The model under review builds one solid part; all positions refer to its coordinate system, in mm. A direction names the side the tool comes from. Round coordinates to 2 decimals unless told otherwise and drop trailing zeros. Order: outer loops, then holes, each group sorted by start corner. A loop starts at its lowest first (then second) coordinate and runs counter-clockwise, first axis right, second up. Notation, with made-up numbers: (-27, 75) - (3, 75) arc R16 cw to (3, 88) - close; hole circle Ø7 at (56.5, -3.75). An arc over 180 degrees is marked (long way). One line per question, with ' | ' between items. Start each with the question number.
Item 1: Add section C-C on z = -13. State the section outline as (x, y) points, and give its area (3 significant figures).
Item 2: Add section B-B on x = 36. State the section outline as (y, z) points.
Item 3: Add section D-D on y = 40. State the section outline as (x, z) points.
Item 4: Draft analysis for pull direction Y (two halves, no side actions). For faces 3 (the face through (6.47, 27.98, -6.56)), 4 (the face through (1.43, 94.08, -51.93)), 5 (the face through (101, 52, -19)), 6 (the face through (51.2, 12.6, 4.4)), state which applies: +Y half, -Y half, draft (parallel to the pull), parting line (faces both ways), or undercut.
Item 5: Insertion check: pin 1 Ø7.5 at (x, y) = (31, 5) entering from -Z; pin 2 Ø3 at (x, y) = (6, 5) entering from +Z; pin 3 Ø1.5 at (x, y) = (23, 18.5) entering from -Z; pin 4 Ø10 at (x, z) = (82.5, -0.5) entering from -Y. Each pin has a flat end and moves straight along its axis. Give the tip position at first contact, or say it passes through.
Item 6: For L1, parallel to Y at x = 60.5, z = -32; L2, parallel to Y at x = 6, z = 1.35; L3, parallel to Z at x = 25, y = 17.5, list the stretches that pass through material, from the lowest coordinate up. Write a range as [from, to].
Item 7: Tool access review of faces 1 (the face through (10.07, 23.49, 17.67)), 2 (the face through (49.793, 94.212, -49.2)): name each direction out of +Z, -Z, +X, -X, +Y, -Y from which nothing blocks a thin tool from reaching the whole face with its end or side.
Item 8: Add section A-A on y = 19. State the section outline as (x, z) points, and give its area (3 significant figures).
from build123d import *

# Parameters (mm, degrees)
SKETCH_1_W               = 101
SKETCH_1_H               = 15
SKETCH_1_R               = 1.55
EXTRUDE_1_DEPTH          = 3
EXTRUDE_2_DEPTH          = 101
FILLET_1_R               = 10
FILLET_2_R               = 5
SKETCH_3_W               = 101
SKETCH_3_H               = 3
EXTRUDE_3_DEPTH          = 41
SKETCH_4_R               = 1.55
CUT_EXTRUDE_1_DEPTH      = 153.872823645
CUT_EXTRUDE_2_DEPTH      = 149.186409795
CUT_EXTRUDE_2_DEPTH_BACK = 10
SKETCH_5_R               = 1.55
CHAMFER_1_SIZE           = 1.4


with BuildPart() as part:
    # 草图1 → 凸台-拉伸1 (new body)
    with BuildSketch(Plane.XY):
        with Locations((50.5, 7.5)):
            Rectangle(SKETCH_1_W, SKETCH_1_H)
        with Locations((6, 5)):
            Circle(SKETCH_1_R, mode=Mode.SUBTRACT)
        with Locations((95, 5)):
            Circle(SKETCH_1_R, mode=Mode.SUBTRACT)
    extrude(amount=EXTRUDE_1_DEPTH)

    # 草图2 → 凸台-拉伸2 (add)
    with BuildSketch(Plane.ZY):
        Polygon((0, 15), (21.650635095, 27.5), (23.150635095, 24.901923789), (3, 13.267949192), align=None)
    extrude(amount=-EXTRUDE_2_DEPTH)

    # 圆角1
    fillet_1_edges = [part.edges().sort_by_distance(p)[0] for p in [
        (50.5, 13.267949192, 3),
    ]]
    fillet(fillet_1_edges, radius=FILLET_1_R)

    # 圆角2
    fillet_2_edges = [part.edges().sort_by_distance(p)[0] for p in [
        (0, 26.200961894, 22.400635095),
        (101, 26.200961894, 22.400635095),
        (101, 0, 1.5),
        (0, 0, 1.5),
    ]]
    fillet(fillet_2_edges, radius=FILLET_2_R)

    # 草图3 → 凸台-拉伸3 (add)
    with BuildSketch(Plane(origin=(0, 11.25, -6.495190528), x_dir=(1, 0, 0), z_dir=(0, 0.8660254037844364, -0.5000000000000041))):
        with Locations((50.5, -9)):
            Rectangle(SKETCH_3_W, SKETCH_3_H)
    extrude(amount=EXTRUDE_3_DEPTH)

    # 镜向3: part across plane


with BuildPart() as part_1:
    add(part.part)
    add(part.part.mirror(Plane(origin=(0, 46.757041555, -26.995190528), x_dir=(0, 0.500000000000004, 0.8660254037844362), z_dir=(0, 0.8660254037844363, -0.5000000000000041))))

    # 草图4 → 切除-拉伸1 (cut, through all)
    with BuildSketch(Plane(origin=(0, 5.25, 9.09326674), x_dir=(1, 0, 0), z_dir=(0, 0.5000000000000041, 0.8660254037844364))):
        with Locations(Location((6, 78.990381057, 0), (0, 0, 270))):
            Circle(SKETCH_4_R)
        with Locations(Location((6, 53.990381057, 0), (0, 0, 270))):
            Circle(SKETCH_4_R)
        with Locations(Location((6, 28.990381057, 0), (0, 0, 270))):
            Circle(SKETCH_4_R)
        with Locations(Location((95, 78.990381057, 0), (0, 0, 270))):
            Circle(SKETCH_4_R)
        with Locations(Location((95, 53.990381057, 0), (0, 0, 270))):
            Circle(SKETCH_4_R)
        with Locations(Location((95, 28.990381057, 0), (0, 0, 270))):
            Circle(SKETCH_4_R)
    extrude(amount=-CUT_EXTRUDE_1_DEPTH, mode=Mode.SUBTRACT)

    # 草图5 → 切除-拉伸2 (cut, two sides: drawn at the far end of the back side and taken through both)
    with BuildSketch(Plane(origin=(0, 82.26408311, -47.495190528), x_dir=(1, 0, 0), z_dir=(0, -0.8660254037844376, 0.500000000000002)).offset(-CUT_EXTRUDE_2_DEPTH_BACK)):
        with Locations(Location((10, 25.5, 0), (0, 0, 270))):
            Circle(SKETCH_5_R)
        with Locations(Location((90, 25.5, 0), (0, 0, 270))):
            Circle(SKETCH_5_R)
    extrude(amount=CUT_EXTRUDE_2_DEPTH + CUT_EXTRUDE_2_DEPTH_BACK, mode=Mode.SUBTRACT)

    # 倒角1
    chamfer_1_edges = [part_1.edges().sort_by_distance(p)[0] for p in [
        (6, 31.698745836, -6.176923789),
        (6, 53.349380931, -18.676923789),
        (95, 53.349380931, -18.676923789),
        (95, 75.000016026, -31.176923789),
        (95, 31.698745836, -6.176923789),
        (6, 75.000016026, -31.176923789),
    ]]
    chamfer(chamfer_1_edges, length=CHAMFER_1_SIZE)


solid = part_1.part
Determined:
1) outline: (0, 37.52) - (101, 37.52) - (101, 43.52) - (0, 43.52) - close | area: 606 mm2
2) outline: (0, 0) - (15, 0) - (86.01, -41) - (93.51, -53.99) - (96.11, -52.49) - (92.36, -46) arc R10 cw to (92.36, -36) - (101.11, -20.85) - (98.51, -19.35) - (87.51, -38.4) - (16.5, 2.6) - (27.5, 21.65) - (24.9, 23.15) - (16.15, 8) arc R10 cw to (7.49, 3) - (0, 3) - close
3) outline: (0, -14.43) - (101, -14.43) - (101, -10.97) - (0, -10.97) - close
4) face 3: undercut | face 4: +Y half | face 5: draft | face 6: -Y half
5) pin 1: z = 0 | pin 2: through | pin 3: z = -2.45 | pin 4: y = 0
6) L1: [70.43, 76.43], [91.21, 94.67] | L2: [0, 3.45], [6.55, 18.66] | L3: [-1.44, 2.02], [4.33, 10.33]
7) face 1: none | face 2: +X, -X, +Y
8) outline: (0, -2.31) - (101, -2.31) - (101, 1.15) - (0, 1.15) - close; (0, 6.93) - (101, 6.93) - (101, 12.93) - (0, 12.93) - close | area: 956 mm2
